Could you check a few things on this model? Use its own coordinates, in mm. A direction names the side the tool comes from. Coordinates: 2 decimals unless noted, no trailing zeros. Order: outer loops, then holes, each group sorted by start corner. A loop starts at its lowest first (then second) coordinate and runs counter-clockwise, first axis right, second up. Notation, with made-up numbers: (-37.5, 67) - (5.5, 67) arc R22 cw to (5.5, 82) - close; hole circle Ø1 at (-18, 82). An arc over 180 degrees is marked (long way). Answer as a JSON object with one key per item and string values. Group by question number.
(1) Imagine slicing it at B-B, the plane z = -23. Write out the boundary of the cut face in (x, y), and give its area (4 significant figures).
(2) Please list where these lines run through material, in increasing order: probe 1 along Z at (x, y) = (103, -14); probe 2 along Z at (x, y) = (34.5, -46); probe 3 along X at (y, z) = (-27.5, -5).
(3) Imagine slicing it at C-C, the plane x = 102. Write out the boundary of the cut face in (y, z).
(4) Imagine slicing it at A-A, the plane y = -80. Write out the boundary of the cut face in (x, z).
(5) Which directions (+Z, -Z, +X, -X, +Y, -Y) give clear straight access to the entire face, cutting with the end or side of a thin tool? Please do faces 1 (the flat face through (150, -74, -65)), 2 (the flat face through (116, -74, -30)).
(6) Will these pins go through, and if not, where does the flat tip stop? P1, Ø1.5, axis at y = -67, z = -25.5, coming from the +X side; P2, Ø12, axis at x = 76.5, y = -92.5, coming from the +Z side.
from build123d import *

# Parameters (mm, degrees)
F1_DEPTH = 150


with BuildPart() as f1:
    # F0 (on Front) → F1 (new body)
    with BuildSketch(Plane.XZ):
        with BuildLine():
            Line((28.197561, 0), (0, 0))
            Line((0, 0), (0, -100))
            Line((0, -100), (150, -100))
            Line((150, -100), (150, -30))
            Line((150, -30), (80.802439, -30))
            ThreePointArc((80.802439, -30), (74.362315, -28.934751), (68.608224, -25.85248))
            Line((68.608224, -25.85248), (40.391776, -4.14752))
            ThreePointArc((40.391776, -4.14752), (34.637685, -1.065249), (28.197561, 0))
        make_face()
    extrude(amount=F1_DEPTH)


solid = f1.part
Result set:
{
 "1": {"outline": "(0, -150) - (64.9, -150) - (64.9, 0) - (0, 0) - close", "area": "9,735 mm^2"},
 "2": {"probe 1": "z = -100 to -30", "probe 2": "z = -100 to -1.02", "probe 3": "x = 0 to 41.5"},
 "3": {"outline": "(-150, -100) - (0, -100) - (0, -30) - (-150, -30) - close"},
 "4": {"outline": "(0, -100) - (150, -100) - (150, -30) - (80.8, -30) arc R20 cw to (68.61, -25.85) - (40.39, -4.15) arc R20 ccw to (28.2, 0) - (0, 0) - close"},
 "5": {"face 1": "+Z, -Z, +X, +Y, -Y", "face 2": "+Z, +X, +Y, -Y"},
 "6": {"P1": "stops at x = 69.14", "P2": "stops at z = -27.14"}
}
